CAD build for the part. Positions are in the model's coordinates, mm. Give positions to 0.01 mm unless a question says otherwise; leave off trailing zeros. Order: outer loops, then holes, each group sorted by start corner. A loop starts at its lowest first (then second) coordinate and runs counter-clockwise, first axis right, second up.
Item 1: Wall check: L1, parallel to Z at x = 9.5, y = 3.45; L2, parallel to Z at x = -29.5, y = 2.4. Give the ranges that are in metal, low to high.
Item 2: Flat gauge pins, fed straight in: P1, Ø1.2, axis at y = 1.5, z = 30, coming from the -X side; P2, Ø1.2, axis at x = -51, y = 1.5, coming from the -Z side. Where does each tip first touch, or does it go through?
Item 3: Band-saw the part on B-B on z = -15. Give the cut face in (x, y).
Item 4: Band-saw the part on A-A on x = 45.5. Give the cut face in (y, z), plus the area to 3 significant figures.
Autodesk Inventor part; units mm, degrees
ref_plane "YZ Plane" through (0, 0, 0) normal (1, 0, 0) x (0, 1, 0)
ref_plane "XZ Plane" through (0, 0, 0) normal (0, 1, 0) x (-1, 0, 0)
ref_plane "XY Plane" through (0, 0, 0) normal (0, 0, 1) x (1, 0, 0)
sketch "Sketch1" plane through (0, 0, 0) normal (0, 1, 0) x (-1, 0, 0)
  line L0 (60, 60) -> (-60, 60)
  line L1 (-60, 60) -> (-60, -60)
  line L2 (-60, -60) -> (60, -60)
  line L3 (60, -60) -> (60, 60)
  point P0 (0, 0)
  dimension "d2" = 120
  dimension "d3" = 120
  dimension "d4" = 60
  dimension "d5" = 60
extrude "Extrusion1" add sketch "Sketch1" along normal blind 4
sketch "Sketch2" plane through (-60, 0, -60) normal (-1, 0, 0) x (0, 0, 1)
  line L0 (12, 0) -> (24, 0)
  line L1 (24, 0) -> (24, 4)
  line L2 (24, 4) -> (12, 4)
  line L3 (12, 4) -> (12, 0)
  line L4 (0, 4) -> (120, 4)
  line L5 (0, 0) -> (0, 4)
  point P0 (60, 0)
  dimension "d8" = 12
  dimension "d9" = 4
  dimension "d10" = 0
  dimension "d11" = 12
extrude "Extrusion2" cut sketch "Sketch2" against normal blind 4
pattern_linear "Rectangular Pattern1" count 5 spacing 24 along (0, 0, 1) of "Extrusion2"
sketch "Sketch3" plane through (-56, 0, 60) normal (-1, 0, 0) x (0, 0, 1)
  line L0 (0, 0) -> (-4, 0)
  line L1 (-4, 0) -> (-4, 4)
  line L2 (-4, 4) -> (0, 4)
  line L3 (0, 4) -> (0, 0)
  line L4 (0, 0) -> (0, 4)
  line L5 (0, 4) -> (-120, 4)
  point P0 (-60, 0)
  dimension "d23" = 4
  dimension "d24" = 4
  dimension "d25" = 0
  dimension "d26" = 0
extrude "Extrusion3" add sketch "Sketch3" along normal blind 4
pattern_circular "Circular Pattern3" count 4 over 360 about axis through (0, -10, 0) along (0, 1, 0) of "Extrusion3", "Extrusion2", "Rectangular Pattern1"
sketch "Sketch4" plane through (0, 4, 0) normal (0, 1, 0) x (1, 0, 0)
  line L0 (-48, 56) -> (-56, 56)
  line L1 (-56, 56) -> (-56, 60)
  line L2 (-60, 60) -> (-56, 60)
  line L3 (-60, 60) -> (-60, 48)
  line L4 (-60, 48) -> (-56, 48)
  line L5 (-56, 48) -> (-56, 36)
  line L6 (-56, 36) -> (-60, 36)
  line L7 (-60, 36) -> (-60, 24)
  line L8 (-60, 24) -> (-56, 24)
  line L9 (-56, 24) -> (-56, 12)
  line L10 (-56, 12) -> (-60, 12)
  line L11 (-60, 12) -> (-60, 0)
  line L12 (-60, 0) -> (-56, 0)
  line L13 (-56, 0) -> (-56, -12)
  line L14 (-56, -12) -> (-60, -12)
  line L15 (-60, -12) -> (-60, -24)
  line L16 (-60, -24) -> (-56, -24)
  line L17 (-56, -24) -> (-56, -36)
  line L18 (-56, -36) -> (-60, -36)
  line L19 (-60, -36) -> (-60, -48)
  line L20 (-60, -48) -> (-56, -48)
  line L21 (-56, -48) -> (-56, -56)
  line L22 (-56, -56) -> (-60, -56)
  line L23 (-60, -60) -> (-60, -56)
  line L24 (-60, -60) -> (-48, -60)
  line L25 (-48, -60) -> (-48, -56)
  line L26 (-48, -56) -> (-36, -56)
  line L27 (-36, -56) -> (-36, -60)
  line L28 (-36, -60) -> (-24, -60)
  line L29 (-24, -60) -> (-24, -56)
  line L30 (-24, -56) -> (-12, -56)
  line L31 (-12, -56) -> (-12, -60)
  line L32 (-12, -60) -> (0, -60)
  line L33 (0, -60) -> (0, -56)
  line L34 (0, -56) -> (12, -56)
  line L35 (12, -56) -> (12, -60)
  line L36 (12, -60) -> (24, -60)
  line L37 (24, -60) -> (24, -56)
  line L38 (24, -56) -> (36, -56)
  line L39 (36, -56) -> (36, -60)
  line L40 (36, -60) -> (48, -60)
  line L41 (48, -60) -> (48, -56)
  line L42 (48, -56) -> (56, -56)
  line L43 (56, -56) -> (56, -60)
  line L44 (60, -60) -> (56, -60)
  line L45 (60, -60) -> (60, -48)
  line L46 (60, -48) -> (56, -48)
  line L47 (56, -48) -> (56, -36)
  line L48 (56, -36) -> (60, -36)
  line L49 (60, -36) -> (60, -24)
  line L50 (60, -24) -> (56, -24)
  line L51 (56, -24) -> (56, -12)
  line L52 (56, -12) -> (60, -12)
  line L53 (60, -12) -> (60, 0)
  line L54 (60, 0) -> (56, 0)
  line L55 (56, 0) -> (56, 12)
  line L56 (56, 12) -> (60, 12)
  line L57 (60, 12) -> (60, 24)
  line L58 (60, 24) -> (56, 24)
  line L59 (56, 24) -> (56, 36)
  line L60 (56, 36) -> (60, 36)
  line L61 (60, 36) -> (60, 48)
  line L62 (60, 48) -> (56, 48)
  line L63 (56, 48) -> (56, 56)
  line L64 (56, 56) -> (60, 56)
  line L65 (60, 60) -> (60, 56)
  line L66 (60, 60) -> (48, 60)
  line L67 (48, 60) -> (48, 56)
  line L68 (48, 56) -> (36, 56)
  line L69 (36, 56) -> (36, 60)
  line L70 (36, 60) -> (24, 60)
  line L71 (24, 60) -> (24, 56)
  line L72 (24, 56) -> (12, 56)
  line L73 (12, 56) -> (12, 60)
  line L74 (12, 60) -> (0, 60)
  line L75 (0, 60) -> (0, 56)
  line L76 (0, 56) -> (-12, 56)
  line L77 (-12, 56) -> (-12, 60)
  line L78 (-12, 60) -> (-24, 60)
  line L79 (-24, 60) -> (-24, 56)
  line L80 (-24, 56) -> (-36, 56)
  line L81 (-36, 56) -> (-36, 60)
  line L82 (-36, 60) -> (-48, 60)
  line L83 (-48, 60) -> (-48, 56)
  line L84 (-48.11, 60.11) -> (-35.89, 60.11)
  line L85 (-35.89, 60.11) -> (-35.89, 56.11)
  line L86 (-35.89, 56.11) -> (-24.11, 56.11)
  line L87 (-24.11, 56.11) -> (-24.11, 60.11)
  line L88 (-24.11, 60.11) -> (-11.89, 60.11)
  line L89 (-11.89, 60.11) -> (-11.89, 56.11)
  line L90 (-11.89, 56.11) -> (-0.11, 56.11)
  line L91 (-0.11, 56.11) -> (-0.11, 60.11)
  line L92 (-0.11, 60.11) -> (12.11, 60.11)
  line L93 (12.11, 60.11) -> (12.11, 56.11)
  line L94 (12.11, 56.11) -> (23.89, 56.11)
  line L95 (23.89, 56.11) -> (23.89, 60.11)
  line L96 (23.89, 60.11) -> (36.11, 60.11)
  line L97 (36.11, 60.11) -> (36.11, 56.11)
  line L98 (36.11, 56.11) -> (47.89, 56.11)
  line L99 (47.89, 56.11) -> (47.89, 60.11)
  line L100 (47.89, 60.11) -> (60.11, 60.11)
  line L101 (60.11, 60.11) -> (60.11, 55.89)
  line L102 (60.11, 55.89) -> (56.11, 55.89)
  line L103 (56.11, 55.89) -> (56.11, 48.11)
  line L104 (56.11, 48.11) -> (60.11, 48.11)
  line L105 (60.11, 48.11) -> (60.11, 35.89)
  line L106 (60.11, 35.89) -> (56.11, 35.89)
  line L107 (56.11, 35.89) -> (56.11, 24.11)
  line L108 (56.11, 24.11) -> (60.11, 24.11)
  line L109 (60.11, 24.11) -> (60.11, 11.89)
  line L110 (60.11, 11.89) -> (56.11, 11.89)
  line L111 (56.11, 11.89) -> (56.11, 0.11)
  line L112 (56.11, 0.11) -> (60.11, 0.11)
  line L113 (60.11, 0.11) -> (60.11, -12.11)
  line L114 (60.11, -12.11) -> (56.11, -12.11)
  line L115 (56.11, -12.11) -> (56.11, -23.89)
  line L116 (56.11, -23.89) -> (60.11, -23.89)
  line L117 (60.11, -23.89) -> (60.11, -36.11)
  line L118 (60.11, -36.11) -> (56.11, -36.11)
  line L119 (56.11, -36.11) -> (56.11, -47.89)
  line L120 (56.11, -47.89) -> (60.11, -47.89)
  line L121 (60.11, -47.89) -> (60.11, -60.11)
  line L122 (60.11, -60.11) -> (55.89, -60.11)
  line L123 (55.89, -60.11) -> (55.89, -56.11)
  line L124 (55.89, -56.11) -> (48.11, -56.11)
  line L125 (48.11, -56.11) -> (48.11, -60.11)
  line L126 (48.11, -60.11) -> (35.89, -60.11)
  line L127 (35.89, -60.11) -> (35.89, -56.11)
  line L128 (35.89, -56.11) -> (24.11, -56.11)
  line L129 (24.11, -56.11) -> (24.11, -60.11)
  line L130 (24.11, -60.11) -> (11.89, -60.11)
  line L131 (11.89, -60.11) -> (11.89, -56.11)
  line L132 (11.89, -56.11) -> (0.11, -56.11)
  line L133 (0.11, -56.11) -> (0.11, -60.11)
  line L134 (0.11, -60.11) -> (-12.11, -60.11)
  line L135 (-12.11, -60.11) -> (-12.11, -56.11)
  line L136 (-12.11, -56.11) -> (-23.89, -56.11)
  line L137 (-23.89, -56.11) -> (-23.89, -60.11)
  line L138 (-23.89, -60.11) -> (-36.11, -60.11)
  line L139 (-36.11, -60.11) -> (-36.11, -56.11)
  line L140 (-36.11, -56.11) -> (-47.89, -56.11)
  line L141 (-47.89, -56.11) -> (-47.89, -60.11)
  line L142 (-47.89, -60.11) -> (-60.11, -60.11)
  line L143 (-60.11, -60.11) -> (-60.11, -55.89)
  line L144 (-60.11, -55.89) -> (-56.11, -55.89)
  line L145 (-56.11, -55.89) -> (-56.11, -48.11)
  line L146 (-56.11, -48.11) -> (-60.11, -48.11)
  line L147 (-60.11, -48.11) -> (-60.11, -35.89)
  line L148 (-60.11, -35.89) -> (-56.11, -35.89)
  line L149 (-56.11, -35.89) -> (-56.11, -24.11)
  line L150 (-56.11, -24.11) -> (-60.11, -24.11)
  line L151 (-60.11, -24.11) -> (-60.11, -11.89)
  line L152 (-60.11, -11.89) -> (-56.11, -11.89)
  line L153 (-56.11, -11.89) -> (-56.11, -0.11)
  line L154 (-56.11, -0.11) -> (-60.11, -0.11)
  line L155 (-60.11, -0.11) -> (-60.11, 12.11)
  line L156 (-60.11, 12.11) -> (-56.11, 12.11)
  line L157 (-56.11, 12.11) -> (-56.11, 23.89)
  line L158 (-56.11, 23.89) -> (-60.11, 23.89)
  line L159 (-60.11, 23.89) -> (-60.11, 36.11)
  line L160 (-60.11, 36.11) -> (-56.11, 36.11)
  line L161 (-56.11, 36.11) -> (-56.11, 47.89)
  line L162 (-56.11, 47.89) -> (-60.11, 47.89)
  line L163 (-60.11, 47.89) -> (-60.11, 60.11)
  line L164 (-60.11, 60.11) -> (-55.89, 60.11)
  line L165 (-55.89, 60.11) -> (-55.89, 56.11)
  line L166 (-55.89, 56.11) -> (-48.11, 56.11)
  line L167 (-48.11, 56.11) -> (-48.11, 60.11)
  point P0 (0, 0)
  dimension "d32" = 0.11
extrude "Extrusion4" add sketch "Sketch4" against normal blind 4 contours L83 L82 L81 L80 L79 L78 L77 L76 L75 L74 L73 L72 L71 L70 L69 L68 L67 L66 L65 L64 L63 L62 L61 L60 L59 L58 L57 L56 L55 L54 L53 L52 L51 L50 L49 L48 L47 L46 L45 L44 L43 L42 L41 L40 L39 L38 L37 L36 L35 L34 L33 L32 L31 L30 L29 L28 L27 L26 L25 L24 L23 L22 L21 L20 L19 L18 L17 L16 L15 L14 L13 L12 L11 L10 L9 L8 L7 L6 L5 L4 L3 L2 L1 L0 | L84 L85 L86 L87 L88 L89 L90 L91 L92 L93 L94 L95 L96 L97 L98 L99 L100 L101 L102 L103 L104 L105 L106 L107 L108 L109 L110 L111 L112 L113 L114 L115 L116 L117 L118 L119 L120 L121 L122 L123 L124 L125 L126 L127 L128 L129 L130 L131 L132 L133 L134 L135 L136 L137 L138 L139 L140 L141 L142 L143 L144 L145 L146 L147 L148 L149 L150 L151 L152 L153 L154 L155 L156 L157 L158 L159 L160 L161 L162 L163 L164 L165 L166 L167
sketch "Sketch5" plane through (0, 0, 0) normal (0, -1, 0) x (1, 0, 0)
  line L0 (-55.89, -56.11) -> (-48.11, -56.11)
  line L1 (-48.11, -56.11) -> (-48.11, -60.11)
  line L2 (-48.11, -60.11) -> (-35.89, -60.11)
  line L3 (-35.89, -60.11) -> (-35.89, -56.11)
  line L4 (-35.89, -56.11) -> (-24.11, -56.11)
  line L5 (-24.11, -56.11) -> (-24.11, -60.11)
  line L6 (-24.11, -60.11) -> (-11.89, -60.11)
  line L7 (-11.89, -60.11) -> (-11.89, -56.11)
  line L8 (-11.89, -56.11) -> (-0.11, -56.11)
  line L9 (-0.11, -56.11) -> (-0.11, -60.11)
  line L10 (-0.11, -60.11) -> (12.11, -60.11)
  line L11 (12.11, -60.11) -> (12.11, -56.11)
  line L12 (12.11, -56.11) -> (23.89, -56.11)
  line L13 (23.89, -56.11) -> (23.89, -60.11)
  line L14 (23.89, -60.11) -> (36.11, -60.11)
  line L15 (36.11, -60.11) -> (36.11, -56.11)
  line L16 (36.11, -56.11) -> (47.89, -56.11)
  line L17 (47.89, -56.11) -> (47.89, -60.11)
  line L18 (47.89, -60.11) -> (60.11, -60.11)
  line L19 (60.11, -60.11) -> (60.11, -55.89)
  line L20 (60.11, -55.89) -> (56.11, -55.89)
  line L21 (56.11, -55.89) -> (56.11, -48.11)
  line L22 (56.11, -48.11) -> (60.11, -48.11)
  line L23 (60.11, -48.11) -> (60.11, -35.89)
  line L24 (60.11, -35.89) -> (56.11, -35.89)
  line L25 (56.11, -35.89) -> (56.11, -24.11)
  line L26 (56.11, -24.11) -> (60.11, -24.11)
  line L27 (60.11, -24.11) -> (60.11, -11.89)
  line L28 (60.11, -11.89) -> (56.11, -11.89)
  line L29 (56.11, -11.89) -> (56.11, -0.11)
  line L30 (56.11, -0.11) -> (60.11, -0.11)
  line L31 (60.11, -0.11) -> (60.11, 12.11)
  line L32 (60.11, 12.11) -> (56.11, 12.11)
  line L33 (56.11, 12.11) -> (56.11, 23.89)
  line L34 (56.11, 23.89) -> (60.11, 23.89)
  line L35 (60.11, 23.89) -> (60.11, 36.11)
  line L36 (60.11, 36.11) -> (56.11, 36.11)
  line L37 (56.11, 36.11) -> (56.11, 47.89)
  line L38 (56.11, 47.89) -> (60.11, 47.89)
  line L39 (60.11, 47.89) -> (60.11, 60.11)
  line L40 (60.11, 60.11) -> (55.89, 60.11)
  line L41 (55.89, 60.11) -> (55.89, 56.11)
  line L42 (55.89, 56.11) -> (48.11, 56.11)
  line L43 (48.11, 56.11) -> (48.11, 60.11)
  line L44 (48.11, 60.11) -> (35.89, 60.11)
  line L45 (35.89, 60.11) -> (35.89, 56.11)
  line L46 (35.89, 56.11) -> (24.11, 56.11)
  line L47 (24.11, 56.11) -> (24.11, 60.11)
  line L48 (24.11, 60.11) -> (11.89, 60.11)
  line L49 (11.89, 60.11) -> (11.89, 56.11)
  line L50 (11.89, 56.11) -> (0.11, 56.11)
  line L51 (0.11, 56.11) -> (0.11, 60.11)
  line L52 (0.11, 60.11) -> (-12.11, 60.11)
  line L53 (-12.11, 60.11) -> (-12.11, 56.11)
  line L54 (-12.11, 56.11) -> (-23.89, 56.11)
  line L55 (-23.89, 56.11) -> (-23.89, 60.11)
  line L56 (-23.89, 60.11) -> (-36.11, 60.11)
  line L57 (-36.11, 60.11) -> (-36.11, 56.11)
  line L58 (-36.11, 56.11) -> (-47.89, 56.11)
  line L59 (-47.89, 56.11) -> (-47.89, 60.11)
  line L60 (-47.89, 60.11) -> (-60.11, 60.11)
  line L61 (-60.11, 60.11) -> (-60.11, 55.89)
  line L62 (-60.11, 55.89) -> (-56.11, 55.89)
  line L63 (-56.11, 55.89) -> (-56.11, 48.11)
  line L64 (-56.11, 48.11) -> (-60.11, 48.11)
  line L65 (-60.11, 48.11) -> (-60.11, 35.89)
  line L66 (-60.11, 35.89) -> (-56.11, 35.89)
  line L67 (-56.11, 35.89) -> (-56.11, 24.11)
  line L68 (-56.11, 24.11) -> (-60.11, 24.11)
  line L69 (-60.11, 24.11) -> (-60.11, 11.89)
  line L70 (-60.11, 11.89) -> (-56.11, 11.89)
  line L71 (-56.11, 11.89) -> (-56.11, 0.11)
  line L72 (-56.11, 0.11) -> (-60.11, 0.11)
  line L73 (-60.11, 0.11) -> (-60.11, -12.11)
  line L74 (-60.11, -12.11) -> (-56.11, -12.11)
  line L75 (-56.11, -12.11) -> (-56.11, -23.89)
  line L76 (-56.11, -23.89) -> (-60.11, -23.89)
  line L77 (-60.11, -23.89) -> (-60.11, -36.11)
  line L78 (-60.11, -36.11) -> (-56.11, -36.11)
  line L79 (-56.11, -36.11) -> (-56.11, -47.89)
  line L80 (-56.11, -47.89) -> (-60.11, -47.89)
  line L81 (-60.11, -47.89) -> (-60.11, -60.11)
  line L82 (-60.11, -60.11) -> (-55.89, -60.11)
  line L83 (-55.89, -60.11) -> (-55.89, -56.11)
  point P0 (0, 0)
equation "\"d2\" = width"
equation "\"d3\" = height"
equation "\"d8\" = finger"
equation "\"d9\" = thickness"
equation "\"d11\" = finger"
equation "\"d19\" = 2 * finger"
equation "\"d23\" = thickness"
equation "\"d24\" = 0.333333 * finger"
equation "\"d27\" = thickness"
equation "\"d32\" = 0.5 * kerf"
equation "\"d33\" = thickness"
properties part number "Lukt_botn"
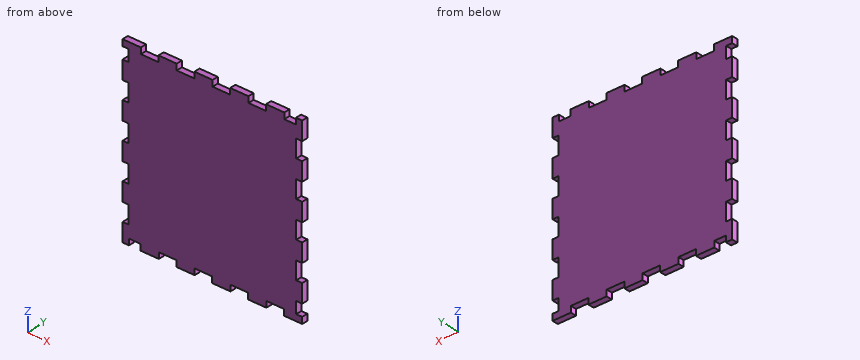
The answers:
1. L1: z = -60.11 to 56.11
1. L2: z = -56.11 to 60.11
2. P1: stops at x = -56.11
2. P2: stops at z = -56.11
3. outline: (-56.11, 0) - (60.11, 0) - (60.11, 4) - (-56.11, 4) - close
4. outline: (0, -56.11) - (4, -56.11) - (4, 60.11) - (0, 60.11) - close
4. area: 465 mm2
